Source: CAD feature listing. Evaluate the final solid. Frame: model axes, mm. A direction names the side the tool comes from. Coordinates: 2 decimals unless noted, no trailing zeros. Write each loop counter-clockwise with the first axis right and the second up, starting at its lowest first coordinate (ties: lowest second). Pieces come first, ordered by that corner, then holes. Notation, with made-up numbers: (61, 84.5) - (102, 84.5) arc R27 cw to (102, 113.5) - close; hole circle Ø5 at (-17.5, 3.25). An arc over 180 degrees is marked (long way). One line per item, written item: value.
from build123d import *

# Parameters (mm, degrees)
SKETCH2_OUTSIDE_W = 37.94
SKETCH2_OUTSIDE_H = 37.94
CUT_EXTRUDE_DEPTH = 23.420400339


with BuildPart() as part:
    # Sketch1 → Base-Extrude (revolve)
    with BuildSketch(Plane.YZ, mode=Mode.PRIVATE) as base_extrude_sk:
        Polygon((0, -2.909378314), (-9.5, -2.909378314), (-14, -0.91417266), (-13.594675009, 0), (-9.5, -1.909378314), (0, -1.909378314), align=None)
    revolve(base_extrude_sk.sketch.rotate(Axis((0, 0, 5.823648763), (0, 0, -1)), 270), axis=Axis((0, 0, 5.823648763), (0, 0, -1)))

    # Sketch2 outside → Cut-Extrude (cut, through all)
    # profile 1 of 2: a face of its own
    with BuildSketch(Plane(origin=(-2.40435344, 1.003568156, -2.909378314), x_dir=(-1, 0, 0), z_dir=(0, 0, -1))):
        with Locations((-2.404, -1.004)):
            Rectangle(SKETCH2_OUTSIDE_W, SKETCH2_OUTSIDE_H)
        with BuildLine():
            Line((-11.712414462, -2.903568156), (-16.274825674, -2.903568156))
            ThreePointArc((-16.274825674, -2.903568156), (-16.40435344, -1.003568156), (-16.274825674, 0.896431844))
            Line((-16.274825674, 0.896431844), (-11.712414462, 0.896431844))
            ThreePointArc((-11.712414462, 0.896431844), (-11.580648789, 1.455212772), (-11.415370745, 2.005014088))
            Line((-11.415370745, 2.005014088), (-15.366534757, 4.286219694))
            ThreePointArc((-15.366534757, 4.286219694), (-14.528709093, 5.996431844), (-13.466534757, 7.577116228))
            Line((-13.466534757, 7.577116228), (-9.515370745, 5.295910622))
            ThreePointArc((-9.515370745, 5.295910622), (-9.121867861, 5.713946265), (-8.703832218, 6.107449149))
            Line((-8.703832218, 6.107449149), (-10.985037824, 10.058613161))
            ThreePointArc((-10.985037824, 10.058613161), (-9.40435344, 11.120787497), (-7.69414129, 11.958613161))
            Line((-7.69414129, 11.958613161), (-5.412935684, 8.007449149))
            ThreePointArc((-5.412935684, 8.007449149), (3.378880136, 6.533288576), (7.07829928, -1.577412552))
            Line((7.07829928, -1.577412552), (11.4852501, -2.758251465))
            ThreePointArc((11.4852501, -2.758251465), (11.118608128, -4.627034788), (10.501737729, -6.428769605))
            Line((10.501737729, -6.428769605), (6.094786909, -5.247930692))
            ThreePointArc((6.094786909, -5.247930692), (5.822887896, -5.753568156), (5.520942513, -6.241858341))
            Line((5.520942513, -6.241858341), (8.74705442, -9.467970247))
            ThreePointArc((8.74705442, -9.467970247), (7.495141497, -10.903063093), (6.060048651, -12.154976016))
            Line((6.060048651, -12.154976016), (2.833936745, -8.928864109))
            ThreePointArc((2.833936745, -8.928864109), (2.34564656, -9.230809492), (1.840009096, -9.502708505))
            Line((1.840009096, -9.502708505), (3.020848009, -13.909659325))
            ThreePointArc((3.020848009, -13.909659325), (1.219113192, -14.526529724), (-0.649670131, -14.893171696))
            Line((-0.649670131, -14.893171696), (-1.830509044, -10.486220876))
            ThreePointArc((-1.830509044, -10.486220876), (-8.187587015, -8.540424889), (-11.712414462, -2.903568156))
        make_face(mode=Mode.SUBTRACT)
    # profile 2 of 2: a face of its own
    with BuildSketch(Plane(origin=(-2.40435344, 1.003568156, -2.909378314), x_dir=(-1, 0, 0), z_dir=(0, 0, -1))):
        with BuildLine():
            Line((-8.471683989, 0.496431844), (-6.65435344, 0.496431844))
            Line((-6.65435344, 0.496431844), (-6.65435344, -2.503568156))
            Line((-6.65435344, -2.503568156), (-8.471683989, -2.503568156))
            ThreePointArc((-8.471683989, -2.503568156), (3.84564656, -1.003568156), (-8.471683989, 0.496431844))
        make_face()
    extrude(amount=-CUT_EXTRUDE_DEPTH, mode=Mode.SUBTRACT)


solid = part.part
1) Draft query along X for faces 5 (the flat face through (11.4, -1.9, -1.4)), 6 (the conical face through (11.519, 0.032, -0.968)), 7 (the conical face through (13.794, 0.027, -0.451)), 8 (the conical face through (5.73, 9.99, -0.97)). Return one class per face: released by +X, released by -X, zero draft, split by the parting line, or undercut.
Values found:
face 5: zero draft
face 6: undercut
face 7: released by +X
face 8: released by -X
2) Section query B-B on x = 0. Output: boundary loops of the cut face in (y, z).
Values found:
outline: (-9.5, -2.91) - (-6.25, -2.91) - (-6.25, -1.91) - (-9.5, -1.91) - close; (6.25, -2.91) - (9.5, -2.91) - (9.5, -1.91) - (6.25, -1.91) - close
3) Reachability of faces 1 (the flat face through (-6.859, -9.546, -1.461)), 2 (the flat face through (-10.713, -4.838, -1.461)), 3 (the flat face through (6, 0, -1.909)), 4 (the flat face through (10.83, 4.06, -1.35)) from +Z, -Z, +X, -X, +Y, -Y: full face, straight path, thin tool, end or side. Return the list, or none.
Values found:
face 1: +Z, -Z, -Y
face 2: +Z, -Z
face 3: +Z
face 4: +Z, -Z, +X
4) Material intervals for line 1 (Y direction, x = 0, z = -2.3); line 2 (X direction, y = 6, z = -0.35); line 3 (Z direction, x = 4.75, y = 8.25), sorted ascending.
Values found:
line 1: -9.5 to -6.25, 6.25 to 9.5
line 2: 11.36 to 12.37
line 3: -2.9 to -1.9
5) Contact query for flat-ended pins moving along their axis: P1, Ø0.8, axis at x = 5, z = -2, coming from the -Y side; P2, Ø5, axis at x = -9.5, y = -10, coming from the -Z side; P3, Ø0.9, axis at x = 11.5, z = -1.5, coming from the -Y side. Output: stop coordinate, or through.
Values found:
P1: y = -8.31
P2: z = -2.11
P3: y = -1.9
6) Section query A-A on y = 0. Output: boundary loops of the cut face in (x, z), then the cut area to 3 significant figures.
Values found:
outline: (-9.5, -2.91) - (-6.25, -2.91) - (-6.25, -1.91) - (-9.5, -1.91) - close; (4.25, -2.91) - (9.5, -2.91) - (14, -0.91) - (13.59, 0) - (9.5, -1.91) - (4.25, -1.91) - close
area: 13.0 mm2
